Part model, mm, in its own coordinate system. Coordinates: 2 decimals unless noted, no trailing zeros. Loops run counter-clockwise (first coordinate to the right, second up) from the corner with the lowest first, then second, coordinate; pieces in that order, holes last. Notation, with made-up numbers: M 11,27.5 L 39,27.5 A20 cw 39,53.5 Z; hole C 49,65 d8. An arc over 180 degrees is marked long. Answer as a JSON object with one key per item and string values. Group by question number.
1. Saw through at A-A on x = 7.5. Write the cut outline in (y, z), then the cut area to 3 significant figures.
2. Saw through at B-B on z = 131. Write the cut outline in (x, y), then the cut area to 3 significant figures.
3. Drop a flat-ended pin along its axis: pin 1 Ø10.5 at (y, z) = (12.7, 12.7) entering from +X. Give the stop position or say it passes through.
4. Drill centre lines: L1, parallel to Y at x = 5.75, z = 169; L2, parallel to Y at x = 24.5, z = 38.1. Where is each one in solid material? Low to high.
from build123d import *

# Parameters (mm, degrees)
SKETCH1_W           = 25.4
SKETCH1_H           = 25.4
SKETCH1_W_2         = 22.225
SKETCH1_H_2         = 22.225
BOSS_EXTRUDE1_DEPTH = 419.1
SKETCH2_R           = 3.2639
CUT_EXTRUDE1_DEPTH  = 421.636577107
CUT_EXTRUDE2_DEPTH  = 421.636577107


with BuildPart() as part:
    # Sketch1 → Boss-Extrude1 (new body)
    with BuildSketch(Plane.XY):
        with Locations((12.7, 12.7)):
            Rectangle(SKETCH1_W, SKETCH1_H)
        with Locations((12.7, 12.7)):
            Rectangle(SKETCH1_W_2, SKETCH1_H_2, mode=Mode.SUBTRACT)
    extrude(amount=BOSS_EXTRUDE1_DEPTH)

    # Sketch2 → Cut-Extrude1 (cut, through all)
    with BuildSketch(Plane.ZY):
        with Locations((12.7, 12.7)):
            Circle(SKETCH2_R)
        with Locations((38.1, 12.7)):
            Circle(SKETCH2_R)
        with Locations((63.5, 12.7)):
            Circle(SKETCH2_R)
        with Locations(Location((355.6, 12.7, 0), (0, 0, 270))):
            Circle(SKETCH2_R)
        with Locations(Location((381, 12.7, 0), (0, 0, 270))):
            Circle(SKETCH2_R)
        with Locations(Location((406.4, 12.7, 0), (0, 0, 270))):
            Circle(SKETCH2_R)
    extrude(amount=-CUT_EXTRUDE1_DEPTH, mode=Mode.SUBTRACT)

    # Sketch3 → Cut-Extrude2 (cut, through all)
    with BuildSketch(Plane(origin=(25.4, 0, 0), x_dir=(0, 0, -1), z_dir=(1, 0, 0))):
        with BuildLine():
            Line((0, 25.4), (0, 0))
            Line((0, 0), (-25.4, 0))
            ThreePointArc((-25.4, 0), (-7.439487758, 7.439487758), (0, 25.4))
        make_face()
    extrude(amount=-CUT_EXTRUDE2_DEPTH, mode=Mode.SUBTRACT)


solid = part.part
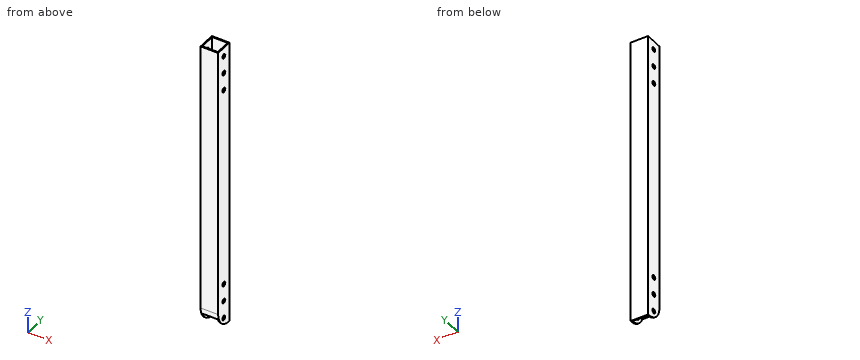
Outcome:
{
 "1": {"outline": "M 0,25.4 A25.4 ccw 1.59,16.56 L 1.59,419.1 L 0,419.1 Z; M 23.81,0.05 A25.4 ccw 25.4,0 L 25.4,419.1 L 23.81,419.1 Z", "area": "1,300 mm²"},
 "2": {"outline": "M 0,0 L 25.4,0 L 25.4,25.4 L 0,25.4 Z; hole M 1.59,1.59 L 23.81,1.59 L 23.81,23.81 L 1.59,23.81 Z", "area": "151 mm²"},
 "3": {"pin 1": "stops at x = 25.4"},
 "4": {"L1": "y = 0 to 1.59, 23.81 to 25.4", "L2": "y = 0 to 9.44, 15.96 to 25.4"}
}
